from build123d import *

# Parameters (mm, degrees)
BOSS_EXTRUDE1_DEPTH = 5.08
SKETCH3_R           = 3.175
BOSS_EXTRUDE2_DEPTH = 7.62
BOSS_EXTRUDE3_START = 2.54
SKETCH6_R           = 5.08
BOSS_EXTRUDE3_DEPTH = 2.54
BOSS_EXTRUDE4_START = 2.54
SKETCH8_R           = 5.08
BOSS_EXTRUDE4_DEPTH = 2.54
CUT_EXTRUDE1_REACH  = 36.454


with BuildPart() as part:
    # Sketch2 → Boss-Extrude1 (new body)
    with BuildSketch(Plane(origin=(0, 0, 0), x_dir=(1, 0, 0), z_dir=(0, 1, 0))):
        with BuildLine():
            Line((-5.08, 25.4), (-5.08, -25.4))
            ThreePointArc((-5.08, -25.4), (0, -30.48), (5.08, -25.4))
            Line((5.08, -25.4), (5.08, 25.4))
            ThreePointArc((5.08, 25.4), (0, 30.48), (-5.08, 25.4))
        make_face()
    extrude(amount=BOSS_EXTRUDE1_DEPTH)

    # Sketch3 → Boss-Extrude2 (add)
    with BuildSketch(Plane(origin=(0, 0, 0), x_dir=(-1, 0, 0), z_dir=(0, -1, 0))):
        with Locations(Location((0, -25.4, 0), (0, 0, 270))):
            Circle(SKETCH3_R)
        with Locations(Location((0, 25.4, 0), (0, 0, 270))):
            Circle(SKETCH3_R)
    extrude(amount=BOSS_EXTRUDE2_DEPTH)

    # Sketch6 → Boss-Extrude3 (add)
    with BuildSketch(Plane.XZ.offset(7.62).offset(BOSS_EXTRUDE3_START)):
        with Locations(Location((0, 25.4, 0), (0, 0, 270))):
            Circle(SKETCH6_R)
    extrude(amount=-BOSS_EXTRUDE3_DEPTH)

    # Sketch8 → Boss-Extrude4 (add)
    with BuildSketch(Plane.XZ.offset(7.62).offset(BOSS_EXTRUDE4_START)):
        with Locations(Location((0, -25.4, 0), (0, 0, 270))):
            Circle(SKETCH8_R)
    extrude(amount=-BOSS_EXTRUDE4_DEPTH)

    # Sketch10 → Cut-Extrude1 (cut, up to next)
    with BuildSketch(Plane(origin=(0, 5.08, 0), x_dir=(1, 0, 0), z_dir=(0, 1, 0)), mode=Mode.PRIVATE) as cut_extrude1_sk1:
        with BuildLine():
            Line((-1.75, 2.121320344), (-1.75, -2.121320344))
            ThreePointArc((-1.75, -2.121320344), (0, -2.75), (1.75, -2.121320344))
            Line((1.75, -2.121320344), (1.75, 2.121320344))
            ThreePointArc((1.75, 2.121320344), (0, 2.75), (-1.75, 2.121320344))
        make_face()
    cut_extrude1_tool1 = extrude(cut_extrude1_sk1.sketch, amount=-CUT_EXTRUDE1_REACH, mode=Mode.PRIVATE) & part.part
    add(cut_extrude1_tool1.solids().sort_by_distance((0, 5.08, 0))[0], mode=Mode.SUBTRACT)


solid = part.part
Read the model definition and answer for the solid it produces. Units are mm, in the model's axes. A direction names the side the tool comes from. Give positions to 0.01 mm unless a question says otherwise; leave off trailing zeros. Loops run counter-clockwise (first coordinate to the right, second up) from the corner with the lowest first, then second, coordinate; pieces in that order, holes last. Notation, with made-up numbers: (33, 56.25) -> (59, 56.25) arc R10 ccw to (59, 68.25) -> close; hole circle Ø10 at (6, 33.5). An arc over 180 degrees is marked (long way). Use a Markdown table: item, result.
Q1. Each of these flat-tipped pins is pushed along its axis until it touches: pin 1 (3 mm diameter, centred on x = -3, z = 8, fed in from -Y); pin 2 (3 mm diameter, centred on x = 2, y = 0.5, fed in from -Z); pin 3 (1 mm diameter, centred on x = -2.5, y = 2, fed in from -Z). Where does it stop, or does it pass through?
Solved:
| item | result |
|---|---|
| pin 1 | stops at y = 0 |
| pin 2 | stops at z = -30.46 |
| pin 3 | stops at z = -30.07 |
Q2. Determine the mould class of faces 6 (the face through (0.03, 2.58, -2.75)), 7 (the face through (0, -7.62, 22)), 8 (the face through (0.223, -8.908, 30.475)) for opening direction X: pulls with the +X half, pulls with the -X half, needs draft (parallel to the pull), parting line crosses it, or undercut.
Solved:
| item | result |
|---|---|
| face 6 | undercut |
| face 7 | needs draft |
| face 8 | parting line crosses it |
Q3. Section A-A, the plane x = 0 is taken. Determine the outline of the cut face in (y, z) (3 decimals), then the cut area to 3 significant figures.
Solved:
| item | result |
|---|---|
| outline | (-10.16, -30.48) -> (-7.62, -30.48) -> (-7.62, -28.575) -> (0, -28.575) -> (0, -30.48) -> (5.08, -30.48) -> (5.08, -2.75) -> (0, -2.75) -> (0, -22.225) -> (-7.62, -22.225) -> (-7.62, -20.32) -> (-10.16, -20.32) -> close; (-10.16, 20.32) -> (-7.62, 20.32) -> (-7.62, 22.225) -> (0, 22.225) -> (0, 2.75) -> (5.08, 2.75) -> (5.08, 30.48) -> (0, 30.48) -> (0, 28.575) -> (-7.62, 28.575) -> (-7.62, 30.48) -> (-10.16, 30.48) -> close |
| area | 430 mm^2 |
Q4. Section C-C, the plane y = 2 is taken. Determine the outline of the cut face in (x, z), then the cut area to 3 significant figures.
Solved:
| item | result |
|---|---|
| outline | (-5.08, -25.4) arc R5.08 ccw to (5.08, -25.4) -> (5.08, 25.4) arc R5.08 ccw to (-5.08, 25.4) -> close; hole (-1.75, -2.12) arc R2.75 ccw to (1.75, -2.12) -> (1.75, 2.12) arc R2.75 ccw to (-1.75, 2.12) -> close |
| area | 579 mm^2 |
Q5. Find the intervals of material crossed by line 1 along Z through (x, y) = (0.25, 3.25); line 2 along Y through (x, z) = (3.5, 13.5); line 3 along Z through (x, y) = (-2, -2.5), in increasing order.
Solved:
| item | result |
|---|---|
| line 1 | z = -30.47 to -2.74, 2.74 to 30.47 |
| line 2 | y = 0 to 5.08 |
| line 3 | z = -27.87 to -22.93, 22.93 to 27.87 |
Q6. Section B-B, the plane z = 1 is taken. Determine the outline of the cut face in (x, y), then the cut area to 3 significant figures.
Solved:
| item | result |
|---|---|
| outline | (-5.08, 0) -> (-1.75, 0) -> (-1.75, 5.08) -> (-5.08, 5.08) -> close; (1.75, 0) -> (5.08, 0) -> (5.08, 5.08) -> (1.75, 5.08) -> close |
| area | 33.8 mm^2 |
Q7. A tool of negligible diameter and unlimited length cuts with its end or side. For faces 1 (the face through (-3.09, -8.91, -21.37)), 2 (the face through (-0.95, -3.76, -22.37)), 3 (the face through (0, -10.16, 25)), 4 (the face through (-1.75, 3, 0)), 5 (the face through (2, 5.08, 0)), from which of +Z, -Z, +X, -X, +Y, -Y can it reach the whole face along a straight path? Write none if from no direction.
Solved:
| item | result |
|---|---|
| face 1 | -Y |
| face 2 | none |
| face 3 | +Z, -Z, +X, -X, -Y |
| face 4 | +Y, -Y |
| face 5 | +Z, -Z, +X, -X, +Y |
Q8. Section D-D, the plane y = -1.25 is taken. Determine the outline of the cut face in (x, z) (3 decimals), then the cut area to 3 significant figures.
Solved:
| item | result |
|---|---|
| outline | circle Ø6.35 at (0, -25.4); circle Ø6.35 at (0, 25.4) |
| area | 63.3 mm^2 |
